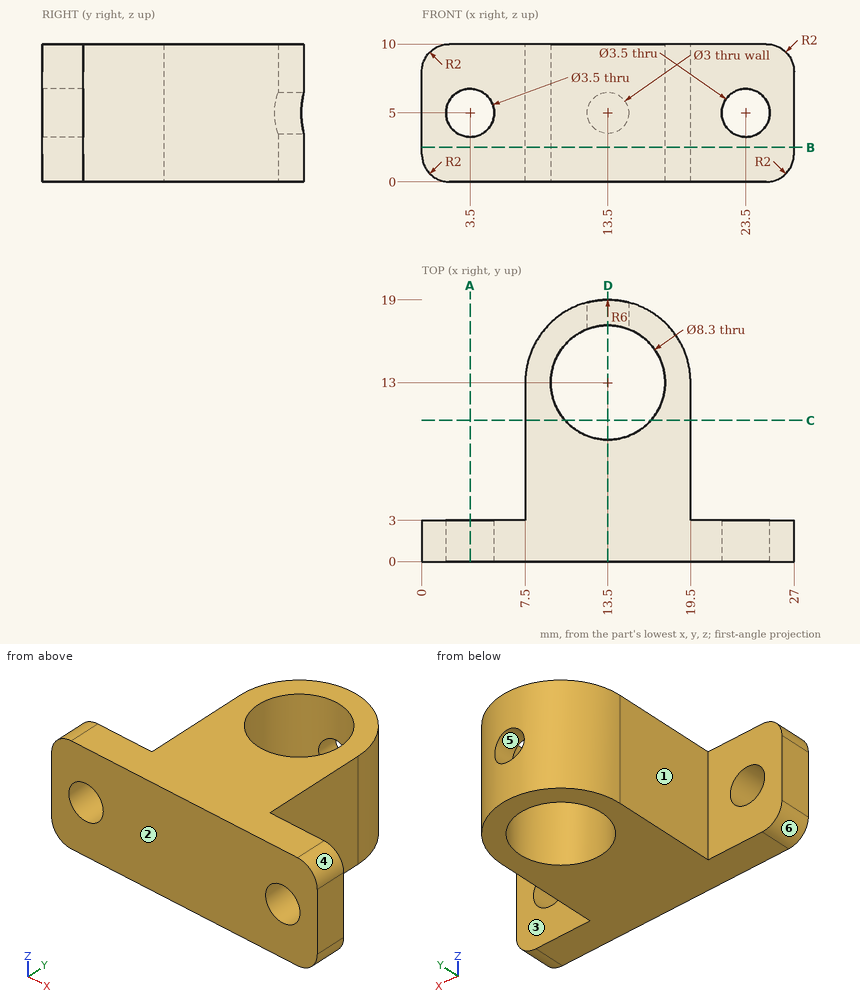
Drawing for the job (mm, zero at the part's lowest x, y, z). A direction names the side the tool comes from. Give positions to 0.01 mm unless a question says otherwise; leave off trailing zeros. Loops run counter-clockwise (first coordinate to the right, second up) from the corner with the lowest first, then second, coordinate; pieces in that order, holes last. Notation, with made-up numbers: (44.5, -40) - (48.5, -40) arc R22 cw to (48.5, -20) - close; hole circle Ø6 at (-12, 4). An arc over 180 degrees is marked (long way). Write item = value, one per line. Start each with the question number.
1) Pull direction Z, two halves, no side cores. Call the marked faces 4, 5 and 6: +Z half, -Z half, draft (parallel to the pull), parting line (faces both ways), or undercut.
2) Band-saw the part on D-D on x = 13.5. Give the cut face in (y, z), plus the area to 3 significant figures.
3) Probe probe 1 along Z at (x, y) = (23.5, 2.35); probe 2 along X at (y, z) = (13, 4.75); probe 3 along Z at (x, y) = (2.5, 1.5). List the from-to ranges inside material, lowest first. Write a range as from..to.
4) Band-saw the part on A-A on x = 3.5. Give the cut face in (y, z).
5) Tool access for the marked faces 1, 2 and 3: list every direction of +Z, -Z, +X, -X, +Y, -Y with a clear straight run to the whole face (end or side of a thin tool).
6) Drop flat-ended pins along their axis: pin 1 Ø1.5 at (x, y) = (21.5, 14) entering from -Z; pin 2 Ø3 at (y, z) = (9.5, 6) entering from +X; pin 3 Ø1 at (x, z) = (21.5, 6) entering from +Y. Give the stop position or say it passes through.
7) Band-saw the part on B-B on z = 2.5. Give the cut face in (x, y), plus the area to 3 significant figures.
8) Band-saw the part on C-C on y = 10.25. Give the cut face in (x, z), plus the area to 3 significant figures.
Final values:
q1.face_4 = +Z half
q1.face_5 = undercut
q1.face_6 = -Z half
q2.outline = (0, 0) - (8.85, 0) - (8.85, 10) - (0, 10) - close; (17.15, 0) - (19, 0) - (19, 3.5) - (17.15, 3.5) - close; (17.15, 6.5) - (19, 6.5) - (19, 10) - (17.15, 10) - close
q2.area = 101 mm²
q3.probe_1 = 0..3.25, 6.75..10
q3.probe_2 = 7.5..9.35, 17.65..19.5
q3.probe_3 = 0..3.56, 6.44..10
q4.outline = (0, 0) - (3, 0) - (3, 3.25) - (0, 3.25) - close; (0, 6.75) - (3, 6.75) - (3, 10) - (0, 10) - close
q5.face_1 = +Z, -Z, -X, +Y
q5.face_2 = +Z, -Z, +X, -X, -Y
q5.face_3 = +Z, -Z, +X, +Y
q6.pin_1 = through
q6.pin_2 = 19.5
q6.pin_3 = 3
q7.outline = (0, 0) - (27, 0) - (27, 3) - (19.5, 3) - (19.5, 13) arc R6 ccw to (7.5, 13) - (7.5, 3) - (0, 3) - close; hole circle Ø8.3 at (13.5, 13)
q7.area = 203 mm²
q8.outline = (7.5, 0) - (10.39, 0) - (10.39, 10) - (7.5, 10) - close; (16.61, 0) - (19.5, 0) - (19.5, 10) - (16.61, 10) - close
q8.area = 57.8 mm²
